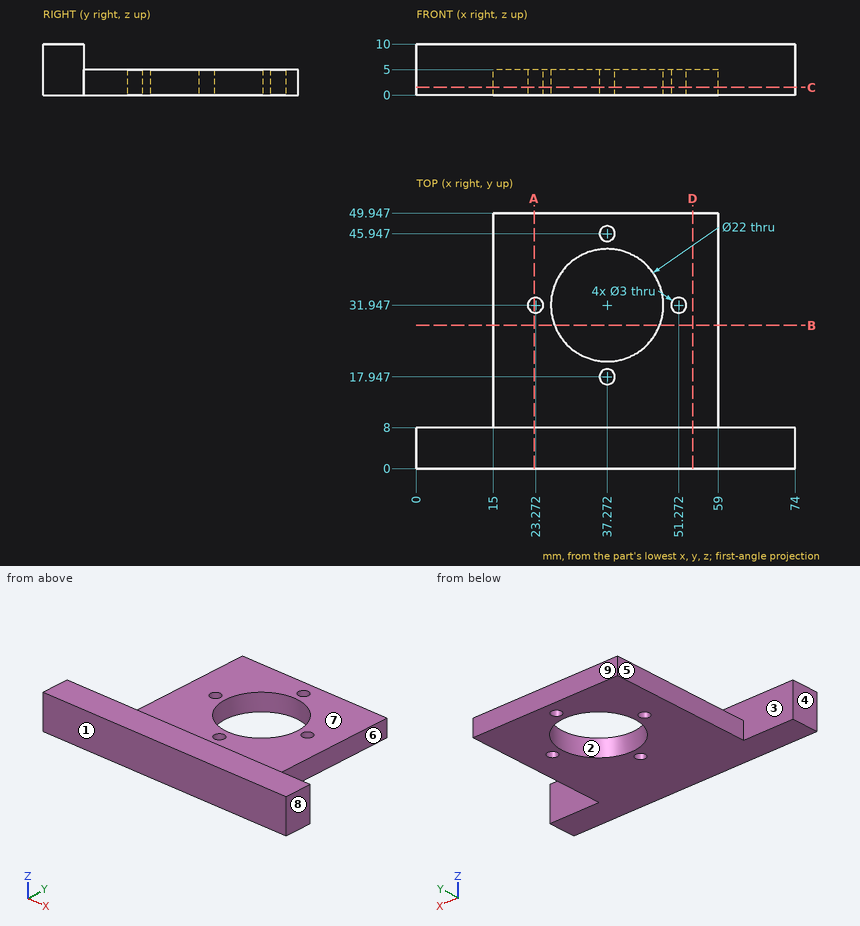
Source: three-view drawing plus pictorial views. Frame: mm from the lowest corner of the part. A direction names the side the tool comes from. Round coordinates to 2 decimals unless told otherwise and drop trailing zeros. Loops run counter-clockwise (first coordinate to the right, second up) from the corner with the lowest first, then second, coordinate; pieces in that order, holes last.
1. Section query D-D on x = 54. Output: boundary loops of the cut face in (y, z).
2. Section query B-B on y = 28. Output: boundary loops of the cut face in (x, z), and give its area (3 significant figures).
3. Ray query, L1, parallel to Z at x = 58, y = 40; L2, parallel to Y at x = 16.5, z = 9.75; L3, parallel to X at y = 40, z = 3.5 (1 decimal). Return the intervals inside material, ascending.
4. Section query C-C on z = 1.5. Output: boundary loops of the cut face in (x, y), and give its area (3 significant figures).
5. Access query for the marked faces 5, 6, 7, 8 and 9. Directions: +Z, -Z, +X, -X, +Y, -Y. A direction counts if a zero-diameter tool reaches every point of the face in a straight line with its end or side. Return the directions, or none.
6. Contact query for flat-ended pins moving along their axis: pin 1 (3.5 mm diameter, centred on x = 51.27, y = 31.95, fed in from -Z); pin 2 (3.5 mm diameter, centred on x = 37.27, y = 17.95, fed in from +Z); pin 3 (5 mm diameter, centred on y = 34.5, z = 1.5, fed in from -X); pin 4 (4 mm diameter, centred on y = 38, z = 2, fed in from +X). Output: stop coordinate, or through.
7. Section query A-A on x = 23. Output: boundary loops of the cut face in (y, z), and give its area (3 significant figures).
8. Mould query, pull axis Y, two halves, no side actions, for the marked faces 1, 2, 3 and 4. Classes: released by +Y, released by -Y, zero draft, split by the parting line, or undercut.
Answers below:
1. outline: (0, 0) - (49.95, 0) - (49.95, 5) - (8, 5) - (8, 10) - (0, 10) - close
2. outline: (15, 0) - (27, 0) - (27, 5) - (15, 5) - close; (47.54, 0) - (59, 0) - (59, 5) - (47.54, 5) - close
2. area: 117 mm2
3. L1: z = 0 to 5
3. L2: y = 0 to 8
3. L3: x = 15 to 29.8, 44.8 to 59
4. outline: (0, 0) - (74, 0) - (74, 8) - (59, 8) - (59, 49.95) - (15, 49.95) - (15, 8) - (0, 8) - close; hole circle Ø3 at (23.27, 31.95); hole circle Ø22 at (37.27, 31.95); hole circle Ø3 at (37.27, 17.95); hole circle Ø3 at (37.27, 45.95); hole circle Ø3 at (51.27, 31.95)
4. area: 2,030 mm2
5. face 5: +Z, -Z, -X, +Y
5. face 6: +Z, -Z, +X, +Y
5. face 7: +Z, +X, -X, +Y
5. face 8: +Z, -Z, +X, +Y, -Y
5. face 9: +Z, -Z, +X, -X, +Y
6. pin 1: stops at z = 0
6. pin 2: stops at z = 5
6. pin 3: stops at x = 15
6. pin 4: stops at x = 59
7. outline: (0, 0) - (30.47, 0) - (30.47, 5) - (8, 5) - (8, 10) - (0, 10) - close; (33.42, 0) - (49.95, 0) - (49.95, 5) - (33.42, 5) - close
7. area: 275 mm2
8. face 1: released by -Y
8. face 2: undercut
8. face 3: released by +Y
8. face 4: zero draft
